Input: part model. Units: mm. Frame: model coordinates. A direction names the side the tool comes from. Give positions to 0.01 mm unless a question says otherwise; leave off trailing zeros. Loops run counter-clockwise (first coordinate to the right, second up) from the corner with the lowest first, then second, coordinate; pieces in that order, holes last. Notation, with made-up numbers: M -27,-26 L -3,-26 A32 cw -3,6 Z; hole C -21,76 d6. An arc over 180 degrees is marked long. Return JSON: item names as keys, results as strings. Group by question number.
Autodesk Inventor part; units mm, degrees
ref_plane "YZ Plane" through (0, 0, 0) normal (1, 0, 0) x (0, 1, 0)
ref_plane "XZ Plane" through (0, 0, 0) normal (0, 1, 0) x (-1, 0, 0)
ref_plane "XY Plane" through (0, 0, 0) normal (0, 0, 1) x (1, 0, 0)
sketch "Sketch1" plane through (0, 0, 0) normal (0, 1, 0) x (-1, 0, 0)
  line L0 (20, 20) -> (20, -20)
  line L1 (20, -20) -> (-20, -20)
  line L2 (-20, -20) -> (-20, 20)
  line L3 (-20, 20) -> (20, 20)
  line L4 (-15, 15) -> (-15, -15) construction
  line L5 (-15, -15) -> (15, -15) construction
  line L6 (15, -15) -> (15, 15) construction
  line L7 (15, 15) -> (-15, 15) construction
  circle A0 centre (15, 15) radius 3.05
  circle A1 centre (15, -15) radius 3.05
  circle A2 centre (-15, -15) radius 3.05
  circle A3 centre (-15, 15) radius 3.05
  line L8 (0, 0) -> (-18.5703, 0) construction
  line L9 (-8, 9) -> (-8, 9)
  line L10 (-10, 11) -> (-12, 11)
  line L11 (-14, 9) -> (-14, -9)
  line L12 (-12, -11) -> (-10, -11)
  line L13 (-8, -9) -> (-8, -9)
  line L14 (8, -9) -> (8, -9)
  line L15 (10, -11) -> (12, -11)
  line L16 (14, -9) -> (14, 9)
  line L17 (12, 11) -> (10, 11)
  line L18 (8, 9) -> (8, 9)
  line L19 (0, 0) -> (0, 18.05) construction
  line L20 (0, 0) -> (-18.05, 0) construction
  arc A4 (-12, 11) -> (-14, 9) centre (-12, 9) ccw
  arc A5 (-8, 9) -> (-10, 11) centre (-10, 9) ccw
  arc A6 (-10, -11) -> (-8, -9) centre (-10, -9) ccw
  arc A7 (-14, -9) -> (-12, -11) centre (-12, -9) ccw
  arc A8 (8, -9) -> (10, -11) centre (10, -9) ccw
  arc A9 (12, -11) -> (14, -9) centre (12, -9) ccw
  arc A10 (14, 9) -> (12, 11) centre (12, 9) ccw
  arc A11 (10, 11) -> (8, 9) centre (10, 9) ccw
  line L21 (8, 9) -> (4, 9)
  line L22 (4, 9) -> (4, 11)
  line L23 (2, 13) -> (-2, 13)
  line L24 (-4, 11) -> (-4, 9)
  line L25 (-4, 9) -> (-8, 9)
  line L26 (-8, -9) -> (-4, -9)
  line L27 (-4, -9) -> (-4, -11)
  line L28 (-2, -13) -> (2, -13)
  line L29 (4, -11) -> (4, -9)
  line L30 (8, -9) -> (4, -9)
  arc A12 (4, 11) -> (2, 13) centre (2, 11) ccw
  arc A13 (-2, 13) -> (-4, 11) centre (-2, 11) ccw
  arc A14 (2, -13) -> (4, -11) centre (2, -11) ccw
  arc A15 (-4, -11) -> (-2, -13) centre (-2, -11) ccw
  point P0 (-8, 11)
  point P1 (-14, 11)
  point P2 (-8, -11)
  point P3 (8, -11)
  point P4 (14, -11)
  point P5 (8, 11)
  point P6 (-4, 13)
  point P7 (-4, -13)
  point P8 (4, -13)
  dimension "d0" = 40
  dimension "d1" = 40
  dimension "d2" = 30
  dimension "d3" = 6.1
  dimension "d53" = 20
  dimension "d54" = 15
  dimension "d57" = 8
  dimension "d58" = 16
  dimension "d59" = 22
  dimension "d60" = 6
  dimension "d61" = 2
  dimension "d96" = 4
  dimension "d97" = 8
  dimension "d98" = 4
  dimension "d99" = 2
extrude "Extrusion5" add sketch "Sketch1" along normal blind 8
sketch "Sketch8" plane through (20, 0, -20) normal (0, 0, -1) x (-1, 0, 0)
  circle A0 centre (20, 4) radius 1.5
  point P0 (20, 0)
  dimension "d100" = 4
  dimension "d101" = 3
sketch "Sketch9" plane through (20, 0, 20) normal (1, 0, 0) x (0, 0, -1)
  line L0 (40, 0) -> (0, 0)
  line L1 (40, 0) -> (40, 8)
  line L2 (0, 8) -> (40, 8)
  line L3 (0, 0) -> (0, 8)
  point P0 (20, 0)
  point P1 (5, 4)
  point P2 (35, 4)
  dimension "d104" = 5
  dimension "d105" = 5
  dimension "d106" = 4
  dimension "d107" = 4
hole "Hole1" at (20, 4, 15) at (20, 4, -15) direction (-1, 0, 0) diameter 2.013 depth 5 tip angle 118
sketch "Sketch10" plane through (-20, 0, -20) normal (-1, 0, 0) x (0, 0, 1)
  circle A0 centre (35, 4) radius 1.0065
  circle A1 centre (5, 4) radius 1.0065
  point P0 (20, 0)
  point P1 (33.9935, 4)
  point P2 (3.9935, 4)
hole "Hole2" at (-20, 4, 15) at (-20, 4, -15) direction (1, 0, 0) diameter 2.013 depth 5 tip angle 118
hole "Hole3" at (0, 4, -20) direction (0, 0, 1) diameter 3.1 end through all
equation "\"d1\" = d0"
properties part number "Holder"
Item 1: Pull-direction query (Y, two-part tool) for faces 4 (the face through (-0.07, 2.45, -16.45)), 5 (the face through (4, 4, 10)); classes: pulls with the +Y half, pulls with the -Y half, needs draft (parallel to the pull), parting line crosses it, or undercut.
Item 2: Section C-C, the plane z = -2. Return loops of the section in (x, y), then the cut area to 3 significant figures.
Item 3: First-contact query: pin 1 Ø10 at (x, z) = (15, 15) entering from +Y. Flat tip, straight axial feed; report the tip coordinate or a pass-through.
Item 4: Section D-D, the plane x = -15. Return loops of the section in (y, z).
Item 5: Reachability of faces 1 (the face through (3.4, 3.94, -12.43)), 2 (the face through (-20, 4, 0)), 3 (the face through (-18.925, 3.956, 13.994)) from +Z, -Z, +X, -X, +Y, -Y: full face, straight path, thin tool, end or side. Return the list, or none.
Item 6: Section B-B, the plane x = 0. Return loops of the section in (y, z), then the cut area to 3 significant figures.
Item 7: Material intervals for line 1 (Z direction, x = -19.05, y = 4); line 2 (Z direction, x = 15, y = 5.25); line 3 (X direction, y = 1.75, z = -8.5), sorted ascending. Write a range as from..to.
Item 8: Section A-A, the plane z = -15. Return loops of the section in (x, y), then the cut area to 3 significant figures.
Answer below:
{
 "1": {"face 4": "undercut", "face 5": "needs draft"},
 "2": {"outline": "M -20,0 L -14,0 L -14,8 L -20,8 Z; M 14,0 L 20,0 L 20,8 L 14,8 Z", "area": "96.0 mm^2"},
 "3": {"pin 1": "y = 8"},
 "4": {"outline": "M 0,-20 L 8,-20 L 8,-18.05 L 0,-18.05 Z; M 0,-11.95 L 8,-11.95 L 8,11.95 L 0,11.95 Z; M 0,18.05 L 8,18.05 L 8,20 L 0,20 Z"},
 "5": {"face 1": "+Y, -Y", "face 2": "+Z, -Z, -X, +Y, -Y", "face 3": "-X"},
 "6": {"outline": "M 0,-20 L 2.45,-20 L 2.45,-13 L 0,-13 Z; M 0,13 L 2.45,13 L 2.45,20 L 0,20 Z; M 5.55,-20 L 8,-20 L 8,-13 L 5.55,-13 Z; M 5.55,13 L 8,13 L 8,20 L 5.55,20 Z", "area": "68.6 mm^2"},
 "7": {"line 1": "-20..-16.01, -13.99..13.99, 16.01..20", "line 2": "-20..-18.05, -11.95..11.95, 18.05..20", "line 3": "-20..-14, 14..20"},
 "8": {"outline": "M -20,0 L -18.05,0 L -18.05,2.99 L -20,2.99 Z; M -20,5.01 L -18.05,5.01 L -18.05,8 L -20,8 Z; M -11.95,0 L 11.95,0 L 11.95,8 L -11.95,8 Z; M 18.05,0 L 20,0 L 20,2.99 L 18.05,2.99 Z; M 18.05,5.01 L 20,5.01 L 20,8 L 18.05,8 Z; hole C 0,4 d3.1", "area": "207 mm^2"}
}
